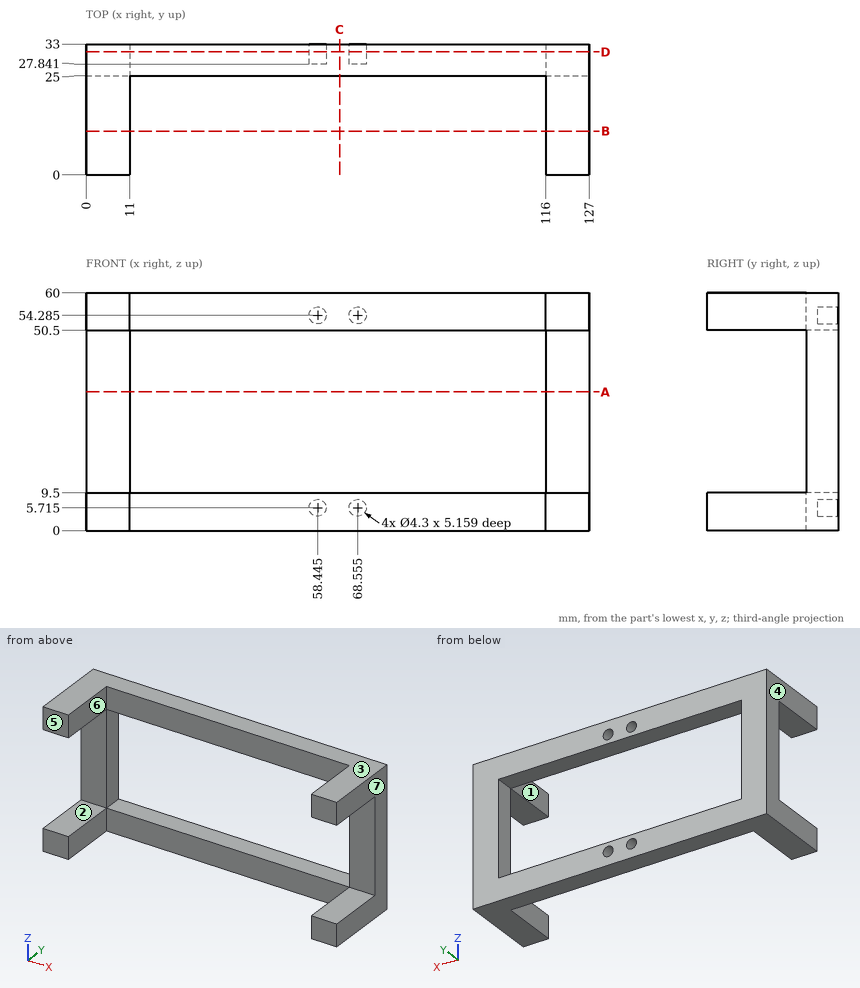
Part print with two shaded views. Sizes in mm from the minimum x, y, z corner. A direction names the side the tool comes from. Coordinates: 2 decimals unless noted, no trailing zeros. Order: outer loops, then holes, each group sorted by start corner. A loop starts at its lowest first (then second) coordinate and runs counter-clockwise, first axis right, second up. Notation, with made-up numbers: (16, 23.5) - (42, 23.5) arc R17 ccw to (42, 30.5) - close; hole circle Ø5 at (1.5, 12.25). An arc over 180 degrees is marked (long way). Write item = value, one per line. Start each with the question number.
1) Saw through at A-A on z = 35. Write the cut outline in (x, y), then the cut area to 3 significant figures.
2) Two-plate mould, pull along X, no slides. Class the marked faces 4, 5, 6 and 7: pulls with the +X half, pulls with the -X half, needs draft (parallel to the pull), parting line crosses it, or undercut.
3) Flat gauge pins, fed straight in: pin 1 Ø2 at (x, z) = (67.5, 5.5) entering from +Y; pin 2 Ø5.5 at (x, z) = (58.445, 5.715) entering from -Y; pin 3 Ø3 at (y, z) = (9, 4.5) entering from -X; pin 4 Ø5 at (y, z) = (5, 13.5) entering from +X. Where does each tip first touch, or does it go through?
4) Saw through at B-B on y = 11. Write the cut outline in (x, z), then the cut area to 3 significant figures.
5) Saw through at C-C on x = 64. Write the cut outline in (y, z).
6) Wall check: line 1 along Z through (x, y) = (110, 29.5); line 2 along X through (y, z) = (27, 41); line 3 along Y through (x, z) = (71.5, 6). Give the ranges that are in metal, low to high. Write a range as from..to.
7) Saw through at D-D on y = 31. Count the separate pieces of the cut face and the enclosed holes in it, then the cut area to 3 significant figures.
8) 3-axis set-ups, long thin cutter, end or side, ignore diameter. For the marked faces 1, 2 and 3: which of +Z, -Z, +X, -X, +Y, -Y reach the whole face in a straight line?
From the geometry:
q1.outline = (0, 25) - (11, 25) - (11, 33) - (0, 33) - close; (116, 25) - (127, 25) - (127, 33) - (116, 33) - close
q1.area = 176 mm^2
q2.face_4 = pulls with the -X half
q2.face_5 = needs draft
q2.face_6 = undercut
q2.face_7 = pulls with the +X half
q3.pin_1 = 27.84
q3.pin_2 = 25
q3.pin_3 = 0
q3.pin_4 = through
q4.outline = (0, 0) - (11, 0) - (11, 9.5) - (0, 9.5) - close; (0, 50.5) - (11, 50.5) - (11, 60) - (0, 60) - close; (116, 0) - (127, 0) - (127, 9.5) - (116, 9.5) - close; (116, 50.5) - (127, 50.5) - (127, 60) - (116, 60) - close
q4.area = 418 mm^2
q5.outline = (25, 0) - (33, 0) - (33, 9.5) - (25, 9.5) - close; (25, 50.5) - (33, 50.5) - (33, 60) - (25, 60) - close
q6.line_1 = 0..9.5, 50.5..60
q6.line_2 = 0..11, 116..127
q6.line_3 = 25..33
q7.separate_pieces = 1
q7.enclosed_holes = 5
q7.area = 3,260 mm^2
q8.face_1 = +Z, -Z, -Y
q8.face_2 = +X, -X, -Y
q8.face_3 = +Z, +X, -X, +Y, -Y
